Here's how the part is built. I have some questions about the finished solid (model axes, mm). Face numbers are marked on the shaded views. Give positions to 0.01 mm unless a question says otherwise; leave off trailing zeros. Write each loop counter-clockwise with the first axis right and the second up, starting at its lowest first coordinate (ties: lowest second). Pieces come first, ordered by that corner, then holes. Notation, with made-up numbers: (80, -3) -> (130, -3) arc R13 ccw to (130, 21) -> close; hole circle Ø3 at (-19, 47). An arc over 180 degrees is marked (long way). Use CSV: the item, a comma, the result in double quotes. Start each with the question number.
(1) Suppose I cut it at B-B on x = 7.5. List the corners of the cut face in (y, z) for me.
(2) For pin 1 Ø12 at (y, z) = (11.5, 10.5) entering from +X; pin 2 Ø0.8 at (x, y) = (3.5, -1) entering from +Z, each with a flat end and sliding along its axis, tell me the tip position at first contact or that it passes through.
(3) Suppose I cut it at A-A on x = 17.2. List the corners of the cut face in (y, z) for me, plus the area to 3 significant figures.
(4) Suppose I cut it at C-C on z = 6.9. Give the number of separate pieces and of enclosed holes in the cut face, plus the area to 3 significant figures.
(5) If we mould it in two halves opening along Y, with no side actions, what happens to the marked faces 1, 2, 3 and 4? For each: pulls with the +Y half, pulls with the -Y half, needs draft (parallel to the pull), parting line crosses it, or undercut.
(6) Suppose I cut it at D-D on x = 11. List the corners of the cut face in (y, z) for me.
(7) I need wall thicknesses on L1, parallel to Z at x = 17.2, y = 22.9; L2, parallel to Y at x = 16, z = 1; L3, parallel to X at y = 8, z = 15. Which ranges of each line are inside material? Lowest first, please. Write a range as [from, to].
from build123d import *

# Parameters (mm, degrees)
F0_W     = 20
F0_H     = 8.6
F1_DEPTH = 1.5
F2_R     = 1.1
F3_DEPTH = 1.5
F4_W     = 2
F4_H     = 20
F5_DEPTH = 12.5


with BuildPart() as f1:
    # F0 (on Front) → F1 (new body)
    with BuildSketch(Plane.XZ):
        with Locations((10, 4.3)):
            Rectangle(F0_W, F0_H)
    extrude(amount=F1_DEPTH)

    # F2 (on face) → F3 (cut, through all)
    with BuildSketch(Plane.XZ.offset(1.5)):
        with Locations((2.8, 6.9)):
            Circle(F2_R)
        with Locations((17.2, 6.9)):
            Circle(F2_R)
        with Locations((2.8, 1.7)):
            Circle(F2_R)
        with Locations((17.2, 1.7)):
            Circle(F2_R)
        with BuildLine():
            Line((14.918079, 8.6), (5.081921, 8.6))
            ThreePointArc((5.081921, 8.6), (10, 6.35), (14.918079, 8.6))
        make_face()
        with BuildLine():
            ThreePointArc((14.918079, 0), (10, 2.25), (5.081921, 0))
            Line((5.081921, 0), (14.918079, 0))
        make_face()
    extrude(amount=-F3_DEPTH, mode=Mode.SUBTRACT)

    # F4 (on face) → F5 (join)
    with BuildSketch(Plane.XZ.offset(1.5)):
        with Locations((-1, 10)):
            Rectangle(F4_W, F4_H)
    extrude(amount=-F5_DEPTH)

    # F7: F1 across plane


with BuildPart() as f1_1:
    add(f1.part)
    add(f1.part.mirror(Plane.XZ.offset(-11)))


solid = f1_1.part
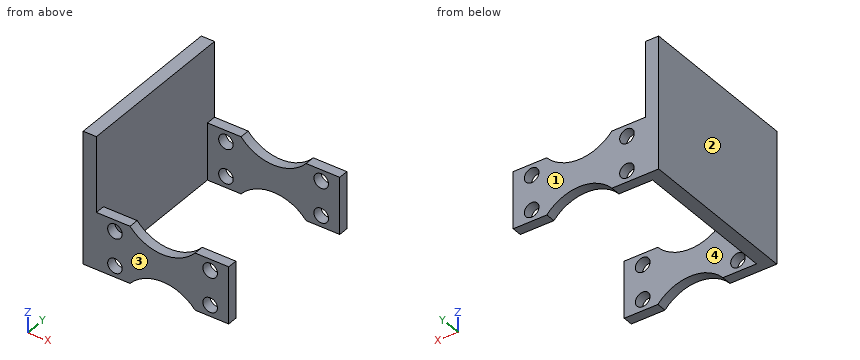
Geometry says:
1,outline,"(-1.5, 1.75) -> (0, 1.75) -> (0, 6.85) -> (-1.5, 6.85) -> close; (22, 1.75) -> (23.5, 1.75) -> (23.5, 6.85) -> (22, 6.85) -> close"
2,pin 1,"x = 0"
2,pin 2,"z = 8.6"
3,outline,"(-1.5, 0) -> (0, 0) -> (0, 0.6) -> (-1.5, 0.6) -> close; (-1.5, 2.8) -> (0, 2.8) -> (0, 5.8) -> (-1.5, 5.8) -> close; (-1.5, 8) -> (0, 8) -> (0, 8.6) -> (-1.5, 8.6) -> close; (22, 0) -> (23.5, 0) -> (23.5, 0.6) -> (22, 0.6) -> close; (22, 2.8) -> (23.5, 2.8) -> (23.5, 5.8) -> (22, 5.8) -> close; (22, 8) -> (23.5, 8) -> (23.5, 8.6) -> (22, 8.6) -> close"
3,area,"12.6 mm²"
4,separate pieces,"7"
4,enclosed holes,"0"
4,area,"81.1 mm²"
5,face 1,"pulls with the +Y half"
5,face 2,"needs draft"
5,face 3,"pulls with the -Y half"
5,face 4,"undercut"
6,outline,"(-1.5, 2.17) -> (0, 2.17) -> (0, 6.43) -> (-1.5, 6.43) -> close; (22, 2.17) -> (23.5, 2.17) -> (23.5, 6.43) -> (22, 6.43) -> close"
7,L1,"[0, 0.6], [2.8, 5.8], [8, 8.6]"
7,L2,"[-1.5, 0], [22, 23.5]"
7,L3,"[-2, 0]"
